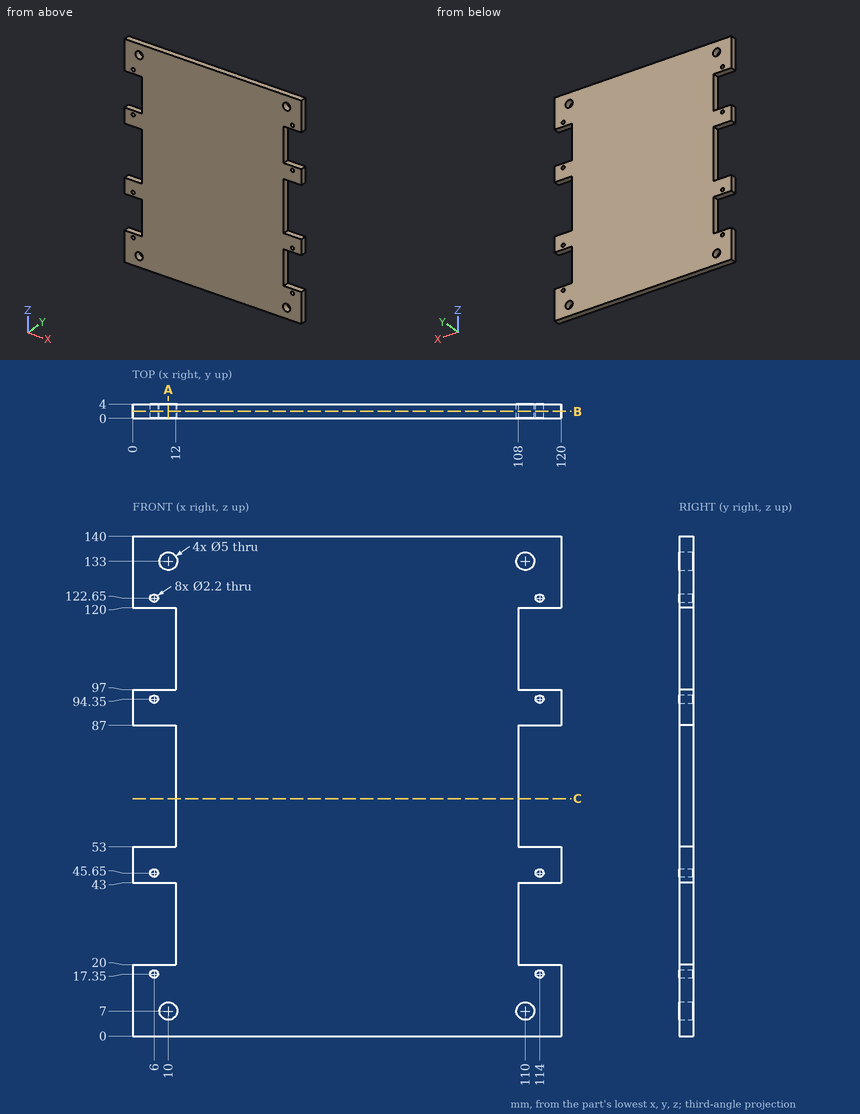
Could you check a few things on this drawing? It's one solid part, dimensions in mm from its lowest x, y, z. Round coordinates to 2 decimals unless told otherwise and drop trailing zeros. Order: outer loops, then holes, each group sorted by start corner. A loop starts at its lowest first (then second) coordinate and runs counter-clockwise, first axis right, second up. Notation, with made-up numbers: M 20.25,11 L 48.25,11 A9 cw 48.25,26 Z; hole C 52,13 d1. An arc over 180 degrees is marked long. Use a Markdown table: item, result.
1) I'm going to push flat-ended pins straight in: P1, Ø1, axis at y = 1, z = 35.5, coming from the -X side; P2, Ø1.2, axis at y = 2.5, z = 35.5, coming from the +X side. Where does each tip first touch, or does it pass through?
Geometry says:
| item | result |
|---|---|
| P1 | stops at x = 12 |
| P2 | stops at x = 108 |
2) Imagine slicing it at A-A (x = 10). List the corners of the cut face in (y, z) for me.
Geometry says:
| item | result |
|---|---|
| outline | M 0,0 L 4,0 L 4,4.5 L 0,4.5 Z; M 0,9.5 L 4,9.5 L 4,20 L 0,20 Z; M 0,43 L 4,43 L 4,53 L 0,53 Z; M 0,87 L 4,87 L 4,97 L 0,97 Z; M 0,120 L 4,120 L 4,130.5 L 0,130.5 Z; M 0,135.5 L 4,135.5 L 4,140 L 0,140 Z |
3) Imagine slicing it at C-C (z = 66.5). List the corners of the cut face in (x, y) for me, then the cut area to 3 significant figures.
Geometry says:
| item | result |
|---|---|
| outline | M 12,0 L 108,0 L 108,4 L 12,4 Z |
| area | 384 mm² |
4) Imagine slicing it at B-B (y = 1.95). Give the number of separate pieces and of enclosed holes in the cut face, then the cut area to 3 significant figures.
Geometry says:
| item | result |
|---|---|
| separate pieces | 1 |
| enclosed holes | 12 |
| area | 14,800 mm² |
5) If I drill on line 1 along X through (y, z) = (1.1, 94.5); line 2 along X through (y, z) = (3.45, 133); line 3 along Z through (x, y) = (110, 1.05), over which ranges is the centre line in solid material (lowest first)?
Geometry says:
| item | result |
|---|---|
| line 1 | x = 0 to 4.91, 7.09 to 112.91, 115.09 to 120 |
| line 2 | x = 0 to 7.5, 12.5 to 107.5, 112.5 to 120 |
| line 3 | z = 0 to 4.5, 9.5 to 20, 43 to 53, 87 to 97, 120 to 130.5, 135.5 to 140 |
